Autodesk Inventor part; units mm, degrees
ref_plane "YZ Plane" through (0, 0, 0) normal (1, 0, 0) x (0, 1, 0)
ref_plane "XZ Plane" through (0, 0, 0) normal (0, 1, 0) x (-1, 0, 0)
ref_plane "XY Plane" through (0, 0, 0) normal (0, 0, 1) x (1, 0, 0)
sketch "Sketch1" plane through (0, 0, 0) normal (0, 0, 1) x (1, 0, 0)
  circle A0 centre (0, 0) radius 4.88
  line L0 (0, 9) -> (32, 9)
  arc A1 (32, -9) -> (32, 9) centre (32, 0) ccw
  line L1 (32, -9) -> (0, -9)
  arc A2 (0, 9) -> (0, -9) centre (0, 0) ccw
  circle A3 centre (32, 0) radius 4.88
  dimension "d0" = 9.76
  dimension "d1" = 9
  dimension "d2" = 32
extrude "Extrusion1" add sketch "Sketch1" along normal blind 3.175
properties part number "tipper_link_A"
Can you work these out from the model? Positions are in its coordinate system, mm. Round coordinates to 2 decimals unless told otherwise and drop trailing zeros. Order: outer loops, then holes, each group sorted by start corner. A loop starts at its lowest first (then second) coordinate and runs counter-clockwise, first axis right, second up. Notation, with made-up numbers: (10.25, -27.75) -> (22.25, -27.75) arc R12 cw to (22.25, -22.75) -> close; hole circle Ø6 at (48.25, -39). An arc over 180 degrees is marked (long way). Return JSON: item names as keys, results as strings. Group by question number.
1. Will this pin go through, and if not, where does the flat tip stop? pin 1 (1 mm diameter, centred on y = -2.5, z = 0.5, fed in from +X).
2. If we section it at D-D, the plane y = -6.5: Write out the boundary of the cut face in (x, z) (3 decimals).
3. If we section it at B-B, the plane z = 1.9: Write out the boundary of the cut face in (x, y).
4. If we section it at A-A, the plane y = 3: Write out the boundary of the cut face in (x, z) (3 decimals).
5. We'd pull the mould along X, two halves only. Please class faces 1 (the face through (41, 0, 2)), 2 (the face through (-9, 0, 2)), 3 (the face through (36.655, -1.466, 1.565)), 4 (the face through (16, 9, 2)): released by +X, released by -X, zero draft, split by the parting line, or undercut.
6. I need wall thicknesses on line 1 (Y direction, x = 32, z = 2); line 2 (X direction, y = 3.5, z = 0.7); line 3 (X direction, y = -4.5, z = 0.8). Which ranges of each line are inside material? Lowest first, please. Write a range as [from, to].
7. If we section it at C-C, the plane y = 0: Write out the boundary of the cut face in (x, z) (3 decimals), then the cut area to 3 significant figures.
Output values:
{
 "1": {"pin 1": "x = 40.77"},
 "2": {"outline": "(-6.225, 0) -> (38.225, 0) -> (38.225, 3.175) -> (-6.225, 3.175) -> close"},
 "3": {"outline": "(0, -9) -> (32, -9) arc R9 ccw to (32, 9) -> (0, 9) arc R9 ccw to start; hole circle Ø9.76 at (0, 0); hole circle Ø9.76 at (32, 0)"},
 "4": {"outline": "(-8.485, 0) -> (-3.849, 0) -> (-3.849, 3.175) -> (-8.485, 3.175) -> close; (3.849, 0) -> (28.151, 0) -> (28.151, 3.175) -> (3.849, 3.175) -> close; (35.849, 0) -> (40.485, 0) -> (40.485, 3.175) -> (35.849, 3.175) -> close"},
 "5": {"face 1": "released by +X", "face 2": "released by -X", "face 3": "undercut", "face 4": "zero draft"},
 "6": {"line 1": "[-9, -4.88], [4.88, 9]", "line 2": "[-8.29, -3.4], [3.4, 28.6], [35.4, 40.29]", "line 3": "[-7.79, -1.89], [1.89, 30.11], [33.89, 39.79]"},
 "7": {"outline": "(-9, 0) -> (-4.88, 0) -> (-4.88, 3.175) -> (-9, 3.175) -> close; (4.88, 0) -> (27.12, 0) -> (27.12, 3.175) -> (4.88, 3.175) -> close; (36.88, 0) -> (41, 0) -> (41, 3.175) -> (36.88, 3.175) -> close", "area": "96.8 mm²"}
}
